Work out the finished part from the listing and answer in its coordinate system (mm). Face numbers are marked on the shaded views. A direction names the side the tool comes from. Round coordinates to 2 decimals unless told otherwise and drop trailing zeros. Write each loop counter-clockwise with the first axis right and the second up, starting at its lowest first coordinate (ties: lowest second). Pieces come first, ordered by that corner, then holes. Notation, with made-up numbers: M 21.5,2.5 L 64.5,2.5 A26 ccw 64.5,36.5 Z; hole C 65,30 d10. An arc over 180 degrees is marked long. One line per item, written item: value. Start each with the question number.
Q1. Find section D-D (x = -2.5). Write down the section's boundary in (y, z) (3 decimals), and give its area (3 significant figures).
Q2. Find section A-A (x = 24.5). Write down the section's boundary in (y, z) (3 decimals), and give its area (3 significant figures).
Q3. The mould has two halves that part along Y. Classify the marked faces 1, 2 and 3: released by +Y, released by -Y, zero draft, split by the parting line, or undercut.
Q4. Given pin 1 Ø0.7 at (x, y) = (40.5, 28) entering from -Z (3 decimals); pin 2 Ø1 at (x, y) = (38.5, 3.5) entering from +Z; pin 3 Ø4 at (x, z) = (37.5, 4) entering from +Y, each flat-ended and moving along its own axis, determine where each tip first touches the part or whether it passes through.
Q5. A tool of negligible diameter and unlimited length cuts with its end or side. For the marked faces 4, 5, 6 and 7, from which of +Z, -Z, +X, -X, +Y, -Y can it reach the whole face along a straight path? Write none if from no direction.
Q6. Find section B-B (z = 1.75). Write down the section's boundary in (x, y) (3 decimals), and give its area (3 significant figures).
Q7. Find section C-C (y = 11). Write down the section's boundary in (x, z) (3 decimals).
Q8. Consider probe 1 along Y at (x, z) = (39.5, 10) (3 decimals); probe 2 along Y at (x, z) = (15, 3.5); probe 3 along Y at (x, z) = (-4, 1.5) (3 decimals). Determine where each line is inside the solid, lowest interval first.
from build123d import *

# Parameters (mm, degrees)
SKETCH1_W           = 38.37
SKETCH1_H           = 35.66
BOSS_EXTRUDE1_DEPTH = 18.93
FILLET1_R           = 0.635
SKETCH3_W           = 17.66
SKETCH3_H           = 2.4
BOSS_EXTRUDE2_DEPTH = 8.74
SKETCH5_R           = 6.015
BOSS_EXTRUDE3_DEPTH = 1
SKETCH7_R           = 2.96
BOSS_EXTRUDE4_DEPTH = 3
SKETCH8_W           = 7.723506563
SKETCH8_H           = 2.58982052
BOSS_EXTRUDE5_DEPTH = 1.27
CUT_EXTRUDE1_REACH  = 54.607


with BuildPart() as part:
    # Sketch1 → Boss-Extrude1 (new body)
    with BuildSketch(Plane.XY):
        with Locations((19.185, 17.83)):
            Rectangle(SKETCH1_W, SKETCH1_H)
    extrude(amount=BOSS_EXTRUDE1_DEPTH)

    # Fillet1
    fillet1_edges = [part.edges().sort_by_distance(p)[0] for p in [
        (38.37, 17.83, 18.93),
        (19.185, 35.66, 18.93),
        (0, 17.83, 18.93),
        (19.185, 35.66, 0),
        (38.37, 17.83, 0),
        (19.185, 0, 0),
        (0, 17.83, 0),
        (0, 35.66, 9.465),
        (38.37, 35.66, 9.465),
        (38.37, 0, 9.465),
        (0, 0, 9.465),
        (19.185, 0, 18.93),
    ]]
    fillet(fillet1_edges, radius=FILLET1_R)

    # Sketch3 → Boss-Extrude2 (add)
    with BuildSketch(Plane.ZY):
        with Locations((9.465, 27.745)):
            Rectangle(SKETCH3_W, SKETCH3_H)
    boss_extrude2 = extrude(amount=BOSS_EXTRUDE2_DEPTH)

    # Sketch5 → Boss-Extrude3 (add)
    with BuildSketch(Plane(origin=(0, 35.66, 0), x_dir=(1, 0, 0), z_dir=(0, 1, 0))):
        with Locations(Location((8.307888536, -9.465, 0), (0, 0, 90))):
            Circle(SKETCH5_R)
    extrude(amount=BOSS_EXTRUDE3_DEPTH)

    # Sketch7 → Boss-Extrude4 (add)
    with BuildSketch(Plane(origin=(0, 36.66, 0), x_dir=(1, 0, 0), z_dir=(0, 1, 0))):
        with Locations(Location((8.307888536, -9.465, 0), (0, 0, 270))):
            Circle(SKETCH7_R)
    extrude(amount=BOSS_EXTRUDE4_DEPTH)

    # Sketch8 → Boss-Extrude5 (add)
    with BuildSketch(Plane(origin=(38.37, 0, 0), x_dir=(0, 0, -1), z_dir=(1, 0, 0))):
        with Locations((-9.516753281, 3.226372892)):
            Rectangle(SKETCH8_W, SKETCH8_H)
    extrude(amount=BOSS_EXTRUDE5_DEPTH)

    # Sketch9 → Cut-Extrude1 (cut, up to next)
    with BuildSketch(Plane(origin=(0, 28.945, 0), x_dir=(1, 0, 0), z_dir=(0, 1, 0)), mode=Mode.PRIVATE) as cut_extrude1_sk1:
        with BuildLine():
            Line((-8.74, -5.094883425), (-7.285254756, -5.094883425))
            ThreePointArc((-7.285254756, -5.094883425), (-4.924130779, -4.445001135), (-7.285253595, -3.795114625))
            Line((-7.285253595, -3.795114625), (-8.74, -3.795114625))
            Line((-8.74, -3.795114625), (-8.74, -5.094883425))
        make_face()
    cut_extrude1_tool1 = extrude(cut_extrude1_sk1.sketch, amount=-CUT_EXTRUDE1_REACH, mode=Mode.PRIVATE) & part.part
    # Sketch9 → Cut-Extrude1 (cut, up to next)
    with BuildSketch(Plane(origin=(0, 28.945, 0), x_dir=(1, 0, 0), z_dir=(0, 1, 0)), mode=Mode.PRIVATE) as cut_extrude1_sk2:
        with BuildLine():
            Line((-8.74, -13.835116616), (-8.74, -15.134883384))
            Line((-8.74, -15.134883384), (-7.285254781, -15.134883384))
            ThreePointArc((-7.285254781, -15.134883384), (-4.924130779, -14.485), (-7.285254781, -13.835116616))
            Line((-7.285254781, -13.835116616), (-8.74, -13.835116616))
        make_face()
    cut_extrude1_tool2 = extrude(cut_extrude1_sk2.sketch, amount=-CUT_EXTRUDE1_REACH, mode=Mode.PRIVATE) & part.part
    cut_extrude1_1 = cut_extrude1_tool1.solids().sort_by_distance((-6.672838, 28.945, 4.445))[0]
    add(cut_extrude1_1, mode=Mode.SUBTRACT)
    cut_extrude1_2 = cut_extrude1_tool2.solids().sort_by_distance((-6.672837, 28.945, 14.485))[0]
    add(cut_extrude1_2, mode=Mode.SUBTRACT)
    cut_extrude1 = cut_extrude1_1 + cut_extrude1_2  # Cut-Extrude1 as one shape, for the pattern or mirror that repeats it

    # Mirror3: Boss-Extrude2, Cut-Extrude1 across plane
    add(boss_extrude2.mirror(Plane.ZY.offset(-19.185)))
    add(cut_extrude1.mirror(Plane.ZY.offset(-19.185)), mode=Mode.SUBTRACT)


solid = part.part
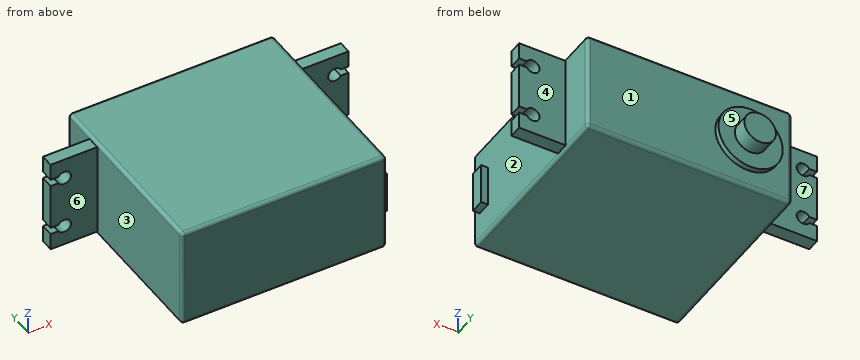
The answers:
1. outline: M 26.545,0.635 L 28.945,0.635 L 28.945,18.295 L 26.545,18.295 Z
1. area: 42.4 mm2
2. outline: M 0,0.635 A0.635 ccw 0.635,0 L 35.025,0 A0.635 ccw 35.66,0.635 L 35.66,18.295 A0.635 ccw 35.025,18.93 L 0.635,18.93 A0.635 ccw 0,18.295 Z
2. area: 675 mm2
3. face 1: released by +Y
3. face 2: undercut
3. face 3: zero draft
4. pin 1: z = 0.635
4. pin 2: z = 18.87
4. pin 3: y = 35.66
5. face 4: +Z, -Z, +X, +Y
5. face 5: +Y
5. face 6: +Z, -Z, -X, -Y
5. face 7: +Z, -Z, -X, +Y
6. outline: M -8.74,26.545 L 0,26.545 L 0,0.635 A0.635 ccw 0.635,0 L 37.735,0 A0.635 ccw 38.37,0.635 L 38.37,26.545 L 47.11,26.545 L 47.11,28.945 L 38.37,28.945 L 38.37,35.025 A0.635 ccw 37.735,35.66 L 0.635,35.66 A0.635 ccw 0,35.025 L 0,28.945 L -8.74,28.945 Z
6. area: 1,410 mm2
7. outline: M 0,0.635 A0.635 ccw 0.635,0 L 37.735,0 A0.635 ccw 38.37,0.635 L 38.37,18.295 A0.635 ccw 37.735,18.93 L 0.635,18.93 A0.635 ccw 0,18.295 Z
8. probe 1: 1.931 to 4.521, 26.545 to 28.945
8. probe 2: 0 to 35.66
8. probe 3: 26.545 to 28.945
